Here's how the part is built. I have some questions about the finished solid (model axes, mm). A direction names the side the tool comes from. Give positions to 0.01 mm unless a question says otherwise; leave off trailing zeros. Loops run counter-clockwise (first coordinate to the right, second up) from the corner with the lowest first, then second, coordinate; pieces in that order, holes last.
Q1. Will these pins go through, and if not, where does the flat tip stop? P1, Ø4, axis at y = 92, z = 11, coming from the +X side; P2, Ø10, axis at x = -57.5, y = 48, coming from the +Z side; P3, Ø5.5, axis at x = 33, z = 10.5, coming from the -Y side.
Q2. If we section it at B-B (y = 45): Please give me the cut outline in (x, z), plus the area to 3 significant figures.
Q3. I need wall thicknesses on line 1 (Y direction, x = 63.5, z = 2.75); line 2 (X direction, y = 74.5, z = 10.5); line 3 (Y direction, x = 65, z = 6.75). Which ranges of each line are inside material? Lowest first, please.
Q4. For faces 1 (the face through (31.5, 96, 10)), 2 (the face through (41.5, 102, 10)), 3 (the face through (36, 64, 10)), 4 (the face through (39, 69, 10)), 5 (the face through (51, 41, 0)), which set-ups out of +Z, -Z, +X, -X, +Y, -Y let a thin tool reach every point of the face, with its end or its side?
Q5. We'd pull the mould along Z, two halves only. Please class faces 6 (the face through (-90, 67, -3.17)), 7 (the face through (39, 96, -2.5)), 8 (the face through (-91, 135, -5)), 9 (the face through (31.5, 72, 10)): +Z half, -Z half, draft (parallel to the pull), parting line (faces both ways), or undercut.
Q6. If we section it at A-A (x = 43.5): Please give me the cut outline in (y, z).
Autodesk Inventor part; units mm, degrees
ref_plane "YZ Plane" through (0, 0, 0) normal (1, 0, 0) x (0, 1, 0)
ref_plane "XZ Plane" through (0, 0, 0) normal (0, 1, 0) x (-1, 0, 0)
ref_plane "XY Plane" through (0, 0, 0) normal (0, 0, 1) x (1, 0, 0)
sketch "Boceto1" plane through (0, 0, 0) normal (0, 1, 0) x (-1, 0, 0)
  line L0 (-98, -7.5) -> (98, -7.5)
  line L1 (98, -7.5) -> (98, 7.5)
  line L2 (98, 7.5) -> (-98, 7.5)
  line L3 (-98, 7.5) -> (-98, -7.5)
  line L4 (-98, -7.5) -> (98, 7.5) construction
  line L5 (98, -7.5) -> (-98, 7.5) construction
  point P0 (0, 0)
  dimension "d0" = 196
  dimension "d1" = 15
extrude "Extrusión1" add sketch "Boceto1" along normal blind 145
sketch "Boceto3" plane through (0, 0, 0) normal (0, -1, 0) x (1, 0, 0)
  line L0 (-98, -7.5) -> (-98, 7.5)
  line L1 (-98, -7.5) -> (-98, 7.5)
  line L2 (-98, 7.5) -> (98, 7.5)
  line L3 (-98, 7.5) -> (98, 7.5)
  line L4 (98, 7.5) -> (98, -7.5)
  line L5 (98, 7.5) -> (98, -7.5)
  line L6 (98, -7.5) -> (-98, -7.5)
  line L7 (98, -7.5) -> (-98, -7.5)
  line L8 (-98, -7.5) -> (-98, 7.5)
  line L9 (98, -7.5) -> (-98, -7.5)
  line L10 (98, 7.5) -> (98, -7.5)
  line L11 (-98, 7.5) -> (98, 7.5)
  line L12 (-98, -7.5) -> (-98, 7.5)
  line L13 (-98, 7.5) -> (98, 7.5)
  line L14 (98, 7.5) -> (98, -7.5)
  line L15 (98, -7.5) -> (-98, -7.5)
  line L16 (-98, -7.5) -> (-98, 7.5)
  line L17 (-98, -7.5) -> (-98, 7.5)
  line L18 (-98, 7.5) -> (98, 7.5)
  line L19 (-98, 7.5) -> (98, 7.5)
  line L20 (98, 7.5) -> (98, -7.5)
  line L21 (98, 7.5) -> (98, -7.5)
  line L22 (98, -7.5) -> (-98, -7.5)
  line L23 (98, -7.5) -> (-98, -7.5)
  line L24 (98, -7.5) -> (-98, -7.5)
  line L25 (-98, -7.5) -> (-98, 7.5)
  line L26 (-98, 7.5) -> (98, 7.5)
  line L27 (98, 7.5) -> (98, -7.5)
  line L28 (98, -7.5) -> (-98, 7.5) construction
  line L29 (-98, -7.5) -> (98, 7.5) construction
  line L30 (90.5, 7.5) -> (90.5, -7.5) construction
  line L31 (88, -7.5) -> (93, -7.5)
  line L32 (88, -7.5) -> (85.5, -3.1699)
  line L33 (85.5, -3.1699) -> (95.5, -3.1699)
  line L34 (95.5, -3.1699) -> (93, -7.5)
  line L35 (0, 7.5) -> (0, -7.5) construction
  line L36 (-88, -7.5) -> (-85.5, -3.1699)
  line L37 (-85.5, -3.1699) -> (-95.5, -3.1699)
  line L38 (-95.5, -3.1699) -> (-93, -7.5)
  point P0 (0, 0)
  point P1 (0, 0)
  point P2 (98, 0)
  dimension "d8" = 7.5
  dimension "d9" = 5
  dimension "d10" = 10
  dimension "d12" = 60
extrude "Extrusión2" cut sketch "Boceto3" against normal blind 135 contours L38 L37 L36 L6 | L32 L33 L34 L6
sketch "Boceto4" plane through (-98, 0, 7.5) normal (0, 0, 1) x (1, 0, 0)
  line L0 (0, 0) -> (0, 145)
  line L1 (0, 45) -> (196, 45) construction
  line L2 (196, 0) -> (196, 145)
  line L3 (0, 0) -> (196, 0)
  line L4 (162, 45) -> (137, 45) construction
  line L5 (162, 49) -> (137, 49)
  line L6 (137, 41) -> (162, 41)
  arc A0 (162, 41) -> (162, 49) centre (162, 45) ccw
  arc A1 (137, 49) -> (137, 41) centre (137, 45) ccw
  line L7 (149.5, 45) -> (149.5, 84) construction
  line L8 (164.5, 69) -> (134.5, 69) construction
  line L9 (134.5, 69) -> (134.5, 99) construction
  line L10 (134.5, 99) -> (164.5, 99) construction
  line L11 (164.5, 99) -> (164.5, 69) construction
  line L12 (164.5, 69) -> (134.5, 99) construction
  line L13 (134.5, 69) -> (164.5, 99) construction
  line L14 (137.5, 72) -> (161.5, 72) construction
  line L15 (161.5, 72) -> (161.5, 96) construction
  line L16 (161.5, 96) -> (137.5, 96) construction
  line L17 (137.5, 96) -> (137.5, 72) construction
  circle A2 centre (161.5, 96) radius 2
  circle A3 centre (137.5, 96) radius 2
  circle A4 centre (161.5, 72) radius 2
  circle A5 centre (137.5, 72) radius 2
  line L18 (134.5, 69) -> (134.5, 79)
  line L19 (134.5, 79) -> (129.5, 79)
  line L20 (129.5, 79) -> (129.5, 64)
  line L21 (129.5, 64) -> (139.5, 64)
  line L22 (139.5, 64) -> (139.5, 69)
  line L23 (139.5, 69) -> (134.5, 69)
  line L24 (149.5, 84) -> (134.5, 84) construction
  line L25 (134.5, 99) -> (134.5, 89)
  line L26 (134.5, 89) -> (129.5, 89)
  line L27 (129.5, 89) -> (129.5, 104)
  line L28 (129.5, 104) -> (139.5, 104)
  line L29 (139.5, 104) -> (139.5, 99)
  line L30 (139.5, 99) -> (134.5, 99)
  line L31 (164.5, 69) -> (164.5, 79)
  line L32 (164.5, 79) -> (169.5, 79)
  line L33 (169.5, 79) -> (169.5, 64)
  line L34 (169.5, 64) -> (159.5, 64)
  line L35 (159.5, 64) -> (159.5, 69)
  line L36 (159.5, 69) -> (164.5, 69)
  line L37 (164.5, 89) -> (169.5, 89)
  line L38 (169.5, 89) -> (169.5, 104)
  line L39 (164.5, 99) -> (164.5, 89)
  line L40 (169.5, 104) -> (159.5, 104)
  line L41 (159.5, 104) -> (159.5, 99)
  line L42 (159.5, 99) -> (164.5, 99)
  point P0 (98, 0)
  point P1 (166, 45)
  dimension "d15" = 45
  dimension "d16" = 8
  dimension "d17" = 25
  dimension "d18" = 30
  dimension "d22" = 39
  dimension "d23" = 30
  dimension "d24" = 30
  dimension "d25" = 3
  dimension "d27" = 4
  dimension "d28" = 4
  dimension "d29" = 4
  dimension "d30" = 4
  dimension "d31" = 10
  dimension "d32" = 5
  dimension "d33" = 5
  dimension "d34" = 5
extrude "Extrusión3" cut sketch "Boceto4" against normal through all contours A0 L6 A1 L5
fillet "Empalme1" radius 0.1 4 edges at (93, 67.5, -7.5) (88, 67.5, -7.5) (-88, 67.5, -7.5) (-93, 67.5, -7.5)
extrude "Extrusión4" cut sketch "Boceto4" against normal blind 10 contours A2 | A3 | A4 | A5
extrude "Extrusión5" add sketch "Boceto4" along normal blind 5 contours L23 L22 L21 L20 L19 L18 | L25 L26 L27 L28 L29 L30 | L31 L32 L33 L34 L35 L36 | L39 L42 L41 L40 L38 L37
equation "\"d27\" = d28"
equation "\"d29\" = d28"
equation "\"d30\" = d28"
properties part number "Tapa_frontal"
Check sheet entries:
1. P1: stops at x = 71.5
1. P2: stops at z = 7.5
1. P3: stops at y = 64
2. outline: (-98, -7.5) - (-93.17, -7.5) arc R0.1 ccw to (-93.09, -7.35) - (-95.5, -3.17) - (-85.5, -3.17) - (-87.91, -7.35) arc R0.1 ccw to (-87.83, -7.5) - (35, -7.5) - (35, 7.5) - (-98, 7.5) - close; (68, -7.5) - (87.83, -7.5) arc R0.1 ccw to (87.91, -7.35) - (85.5, -3.17) - (95.5, -3.17) - (93.09, -7.35) arc R0.1 ccw to (93.17, -7.5) - (98, -7.5) - (98, 7.5) - (68, 7.5) - close
2. area: 2,380 mm2
3. line 1: y = 0 to 41, 49 to 70, 74 to 94, 98 to 145
3. line 2: x = 31.5 to 36.5, 66.5 to 71.5
3. line 3: y = 0 to 41.13, 48.87 to 70.68, 73.32 to 94.68, 97.32 to 145
4. face 1: +Z, -X, +Y, -Y
4. face 2: +Z, +Y, -Y
4. face 3: +Z, +X, -X, -Y
4. face 4: +Z
4. face 5: +Z, -Z
5. face 6: undercut
5. face 7: +Z half
5. face 8: undercut
5. face 9: draft
6. outline: (0, -7.5) - (41, -7.5) - (41, 7.5) - (0, 7.5) - close; (49, -7.5) - (145, -7.5) - (145, 7.5) - (49, 7.5) - close
